Check sheet for the drawn part. Datum: minimum x, y, z corner. Units: mm. A direction names the side the tool comes from. Give positions to 0.01 mm unless a question says otherwise; leave off trailing zeros. Order: outer loops, then holes, each group sorted by start corner. A loop starts at its lowest first (then second) coordinate and runs counter-clockwise, first axis right, second up.
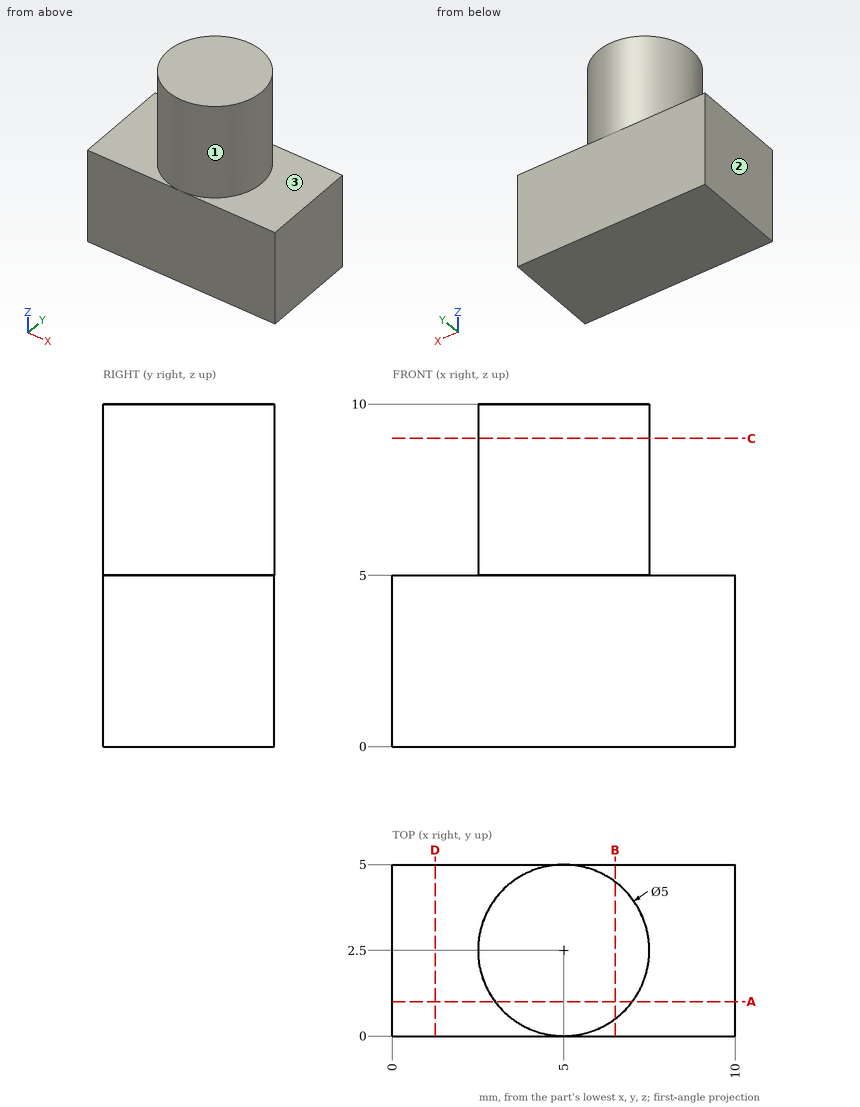
Item 1: Scan lines: L1, parallel to Z at x = 1.25, y = 4.3; L2, parallel to Y at x = 6.75, z = 5.5; L3, parallel to X at y = 1.45, z = 7. Record each from-to range of solid material in increasing order.
Reported:
L1: z = 0 to 5
L2: y = 0.71 to 4.29
L3: x = 2.73 to 7.27
Item 2: Sectioned sample at B-B (x = 6.5). Enter the section's corners in (y, z), and give its area (3 significant figures).
Reported:
outline: (0, 0) - (5, 0) - (5, 5) - (4.5, 5) - (4.5, 10) - (0.5, 10) - (0.5, 5) - (0, 5) - close
area: 45.0 mm2
Item 3: Sectioned sample at C-C (z = 9). Enter the section's corners in (x, y), and give its area (3 significant figures).
Reported:
outline: circle Ø5 at (5, 2.5)
area: 19.6 mm2
Item 4: Set-up check for the marked faces 1, 2 and 3: record each of +Z, -Z, +X, -X, +Y, -Y from which the full face is reachable in a straight line by a thin tool's end or side.
Reported:
face 1: +Z
face 2: +Z, -Z, -X, +Y, -Y
face 3: +Z, +X
Item 5: Gauge pin test, flat end, axial feed: pin 1 (1 mm diameter, centred on x = 3, z = 7, fed in from -Y). Record the tip position at first contact, or that the pin passes through.
Reported:
pin 1: stops at y = 0.5
Item 6: Sectioned sample at A-A (y = 1). Enter the section's corners in (x, z).
Reported:
outline: (0, 0) - (10, 0) - (10, 5) - (7, 5) - (7, 10) - (3, 10) - (3, 5) - (0, 5) - close
Item 7: Sectioned sample at D-D (x = 1.25). Enter the section's corners in (y, z).
Reported:
outline: (0, 0) - (5, 0) - (5, 5) - (0, 5) - close
